```python
from build123d import *

# Parameters (mm, degrees)
F0_R      = 44.358045
F1_DEPTH  = 150
F2_R      = 5.08
F3_R      = 31.478982
F4_DEPTH  = 20
F5_R      = 31.879321
F6_DEPTH  = 10
F7_SIZE   = 5
F8_SIZE   = 5
F9_R      = 5
F10_R     = 31.442334
F11_DEPTH = 25
F12_R     = 31.785479
F13_DEPTH = 25
F14_R     = 32.188515
F15_DEPTH = 25


with BuildPart() as f1:
    # F0 (on Top) → F1 (new body)
    with BuildSketch(Plane.XY):
        Circle(F0_R)
    extrude(amount=F1_DEPTH)

    # F2
    f2_edges = [f1.edges().sort_by_distance(p)[0] for p in [
        (-44.358045, 0, 150),
    ]]
    fillet(f2_edges, radius=F2_R)

    # F3 (on face) → F4 (join)
    with BuildSketch(Plane.XY.offset(150)):
        Circle(F3_R)
    extrude(amount=-F4_DEPTH)

    # F5 (on face) → F6 (cut)
    with BuildSketch(Plane.XY.offset(150)):
        Circle(F5_R)
    extrude(amount=-F6_DEPTH, mode=Mode.SUBTRACT)

    # F7
    f7_edges = [f1.edges().sort_by_distance(p)[0] for p in [
        (-31.879321, 0, 140),
    ]]
    chamfer(f7_edges, length=F7_SIZE)

    # F8
    f8_edges = [f1.edges().sort_by_distance(p)[0] for p in [
        (-26.879321, 0, 140),
    ]]
    chamfer(f8_edges, length=F8_SIZE)

    # F9
    f9_edges = [f1.edges().sort_by_distance(p)[0] for p in [
        (-44.358045, 0, 0),
    ]]
    fillet(f9_edges, radius=F9_R)

    # F10 (on face) → F11 (join)
    with BuildSketch(Plane(origin=(0, 0, 0), x_dir=(1, 0, 0), z_dir=(0, 0, -1))):
        Circle(F10_R)
    extrude(amount=-F11_DEPTH)

    # F12 (on face) → F13 (join)
    with BuildSketch(Plane(origin=(0, 0, 0), x_dir=(1, 0, 0), z_dir=(0, 0, -1))):
        Circle(F12_R)
    extrude(amount=-F13_DEPTH)

    # F14 (on face) → F15 (join)
    with BuildSketch(Plane(origin=(0, 0, 0), x_dir=(1, 0, 0), z_dir=(0, 0, -1))):
        Circle(F14_R)
    extrude(amount=-F15_DEPTH)


solid = f1.part
```
For this review, take the finished solid that the model builds, in its own axes (mm). A direction names the side the tool comes from. Round coordinates to 2 decimals unless told otherwise and drop trailing zeros. Write each loop counter-clockwise with the first axis right and the second up, starting at its lowest first coordinate (ties: lowest second). Pieces come first, ordered by that corner, then holes. Notation, with made-up numbers: (71.5, -3.5) - (120.5, -3.5) arc R30 ccw to (120.5, 23.5) - close; hole circle Ø10 at (11, 42.25). An arc over 180 degrees is marked (long way). Answer as a JSON object with one key per item and string values.
1. For pin 1 Ø22 at (x, y) = (-7.5, 9) entering from +Z; pin 2 Ø1 at (x, y) = (-29.5, 19) entering from -Z; pin 3 Ø10 at (x, y) = (5.5, -12.5) entering from +Z; pin 4 Ø5 at (x, z) = (29.5, 48) entering from -Y, all flat-tipped, find the tip position at first contact; note any pin that passes through.
Response values:
{"pin 1": "stops at z = 140.35", "pin 2": "stops at z = 0", "pin 3": "stops at z = 140", "pin 4": "stops at y = -35.19"}
2. To check wall thickness, follow line 1 along Z through (x, y) = (-6, -0.5); line 2 along Z through (x, y) = (-31, 24.5); line 3 along Y through (x, z) = (0, 146.15). State the ranges of each line that lie inside material, in increasing order.
Response values:
{"line 1": "z = 0 to 140", "line 2": "z = 0 to 149.99", "line 3": "y = -44.21 to -31.88, 31.88 to 44.21"}
3. We need section A-A on x = 0. Give the boundary of the cut face in (y, z), then the cut area to 3 significant figures.
Response values:
{"outline": "(-44.36, 5) arc R5 ccw to (-39.36, 0) - (39.36, 0) arc R5 ccw to (44.36, 5) - (44.36, 144.92) arc R5.08 ccw to (39.28, 150) - (31.88, 150) - (31.88, 145) - (30.41, 143.54) - (21.88, 140) - (-21.88, 140) - (-30.41, 143.54) - (-31.88, 145) - (-31.88, 150) - (-39.28, 150) arc R5.08 ccw to (-44.36, 144.92) - close", "area": "12,700 mm2"}
4. We need section C-C on z = 124. Give the boundary of the cut face in (x, y), then the cut area to 3 significant figures.
Response values:
{"outline": "circle Ø88.72 at (0, 0)", "area": "6,180 mm2"}
5. Tool access review of faces 1 (the face through (14.71, -28.282, 147.535)), 2 (the face through (-0.2, 32.2, 150)): name each direction out of +Z, -Z, +X, -X, +Y, -Y from which nothing blocks a thin tool from reaching the whole face with its end or side.
Response values:
{"face 1": "+Z", "face 2": "+Z, +X, -X, +Y, -Y"}
